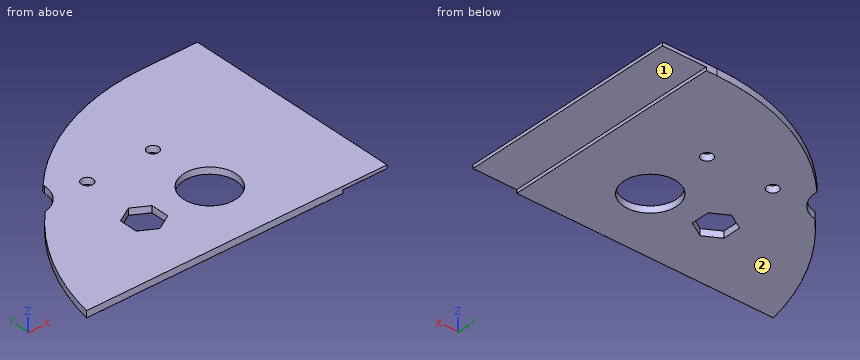
from build123d import *

# Parameters (mm, degrees)
F1_DEPTH  = 3
F3_DEPTH  = 25
F4_R      = 5
F5_R      = 12
F5_R_2    = 2.65
F6_DEPTH  = 25
F7_W      = 78
F7_H      = 55.5
F7_R      = 2
F8_DEPTH  = 25
F9_R      = 8.15
F10_DEPTH = 25
F12_W     = 300.7349916597
F12_H     = 105.2985801398
F13_DEPTH = 25
F14_W     = 20
F14_H     = 100
F15_DEPTH = 1.5
F17_DEPTH = 25
F19_DEPTH = 3


with BuildPart() as f1:
    # F0 (on Top) → F1 (new body)
    with BuildSketch(Plane.XY):
        with BuildLine():
            Line((-197.8147600734, 20.7911690818), (-202.2340594865, 0))
            Line((-202.2340594865, 0), (216.0975214603, 0))
            Line((216.0975214603, 0), (209.2885731253, 20.7911690818))
            ThreePointArc((209.2885731253, 20.7911690818), (167.4870934164, 78.1154778874), (100, 100))
            Line((100, 100), (-100, 100))
            ThreePointArc((-100, 100), (-162.932039105, 77.7145961457), (-197.8147600734, 20.7911690818))
        make_face()
    extrude(amount=F1_DEPTH)

    # F2 (on face) → F3 (cut)
    with BuildSketch(Plane.XY.offset(3)):
        with BuildLine():
            ThreePointArc((1.5842979518, 0), (9.4530988092, 4.1693984068), (12.6, 12.5))
            ThreePointArc((12.6, 12.5), (12.2192388124, 15.5741182224), (11.0999678023, 18.4624420155))
            ThreePointArc((11.0999678023, 18.4624420155), (0, 25.1), (-11.0999678023, 18.4624420155))
            ThreePointArc((-11.0999678023, 18.4624420155), (-11.1999147641, 6.7274867453), (-1.5842979518, 0))
            Line((-1.5842979518, 0), (1.5842979518, 0))
        make_face()
        with BuildLine():
            ThreePointArc((11.0999678023, 18.4624420155), (12.2192388124, 15.5741182224), (12.6, 12.5))
            ThreePointArc((12.6, 12.5), (9.4530988092, 4.1693984068), (1.5842979518, 0))
            Line((1.5842979518, 0), (21.7592636698, 0))
            Line((21.7592636698, 0), (11.0999678023, 18.4624420155))
        make_face()
        with BuildLine():
            ThreePointArc((-1.5842979518, 0), (0, -0.1), (1.5842979518, 0))
            Line((1.5842979518, 0), (-1.5842979518, 0))
        make_face()
        with BuildLine():
            ThreePointArc((-1.5842979518, 0), (-11.1999147641, 6.7274867453), (-11.0999678023, 18.4624420155))
            Line((-11.0999678023, 18.4624420155), (-21.7592636698, 0))
            Line((-21.7592636698, 0), (-1.5842979518, 0))
        make_face()
    extrude(amount=-F3_DEPTH, mode=Mode.SUBTRACT)

    # F4
    f4_edges = [f1.edges().sort_by_distance(p)[0] for p in [
        (-21.759264, 0, 1.5),
        (21.759264, 0, 1.5),
    ]]
    fillet(f4_edges, radius=F4_R)

    # F5 (on face) → F6 (cut)
    with BuildSketch(Plane.XY.offset(3)):
        Polygon((-160, 38.3138438763), (-167.2, 34.1569219382), (-167.2, 25.8430780618), (-160, 21.6861561237), (-152.8, 25.8430780618), (-152.8, 34.1569219382), align=None)
        with Locations((-130, 30)):
            Circle(F5_R)
        with Locations((-130, 60)):
            Circle(F5_R_2)
        with Locations((-160, 60)):
            Circle(F5_R_2)
    extrude(amount=-F6_DEPTH, mode=Mode.SUBTRACT)

    # F7 (on face) → F8 (cut)
    with BuildSketch(Plane.XY.offset(3)):
        with Locations((0, 57.75)):
            Rectangle(F7_W, F7_H)
        with Locations((-42.6313167033, 28.25)):
            Circle(F7_R)
        with Locations((-42.6313167033, 87.25)):
            Circle(F7_R)
        with Locations((42.3686832967, 87.25)):
            Circle(F7_R)
        with Locations((42.3686832967, 28.25)):
            Circle(F7_R)
    extrude(amount=-F8_DEPTH, mode=Mode.SUBTRACT)

    # F9 (on face) → F10 (cut)
    with BuildSketch(Plane.XY.offset(3)):
        with Locations((115, 30)):
            Circle(F9_R)
    extrude(amount=-F10_DEPTH, mode=Mode.SUBTRACT)

    # F12 (on face) → F13 (cut)
    with BuildSketch(Plane.XY.offset(3)):
        with Locations((75.3674958299, 52.6492900699)):
            Rectangle(F12_W, F12_H)
    extrude(amount=-F13_DEPTH, mode=Mode.SUBTRACT)

    # F14 (on face) → F15 (cut)
    with BuildSketch(Plane(origin=(0, 0, 0), x_dir=(1, 0, 0), z_dir=(0, 0, -1))):
        with Locations((-85, -50)):
            Rectangle(F14_W, F14_H)
    extrude(amount=-F15_DEPTH, mode=Mode.SUBTRACT)

    # F16 (on face) → F17 (cut)
    with BuildSketch(Plane.XY.offset(3)):
        with BuildLine():
            ThreePointArc((-183.2262560087, 55.4381665532), (-175.8146533038, 59.7113164576), (-172.8869867134, 67.75))
            ThreePointArc((-172.8869867134, 67.75), (-172.891816845, 68.0974621682), (-172.9063035068, 68.4446558102))
            ThreePointArc((-172.9063035068, 68.4446558102), (-178.3366850582, 62.1559633028), (-183.2262560087, 55.4381665532))
        make_face()
        with BuildLine():
            ThreePointArc((-183.2262560087, 55.4381665532), (-178.3366850582, 62.1559633028), (-172.9063035068, 68.4446558102))
            ThreePointArc((-172.9063035068, 68.4446558102), (-195.1790723457, 75.5194954128), (-183.2262560087, 55.4381665532))
        make_face()
    extrude(amount=-F17_DEPTH, mode=Mode.SUBTRACT)

    # F18 (on face) → F19 (join)
    with BuildSketch(Plane.XY.offset(3)):
        with BuildLine():
            Line((-183.2262560087, 0), (-183.2262560087, 55.4381665532))
            ThreePointArc((-183.2262560087, 55.4381665532), (-201.7549584248, 29.8250444644), (-212.2340594865, 0))
            Line((-212.2340594865, 0), (-183.2262560087, 0))
        make_face()
    extrude(amount=-F19_DEPTH)


solid = f1.part
Can you work these out from the model? Positions are in its coordinate system, mm. Face numbers are marked on the shaded views. A direction names the side the tool comes from. Give positions to 0.01 mm unless a question says otherwise; leave off trailing zeros. Order: outer loops, then holes, each group sorted by start corner. A loop starts at its lowest first (then second) coordinate and runs counter-clockwise, first axis right, second up. Notation, with made-up numbers: M 33.5,76.25 L 72.5,76.25 A28 ccw 72.5,112.25 Z; hole C -27.75,-20.75 d9. An arc over 180 degrees is marked long. Use a Markdown table: item, result. Add a question column.
Item 1: Suppose I cut it at A-A (z = 2). List the corners of the cut face in (x, y) for me.
Item 2: Will these pins go through, and if not, where does the flat tip stop? pin 1 (10 mm diameter, centred on x = -83, y = 58.5, fed in from -Z); pin 2 (4 mm diameter, centred on x = -160, y = 60, fed in from +Z); pin 3 (0.8 mm diameter, centred on y = 70, z = 1, fed in from +X); pin 4 (0.9 mm diameter, centred on y = 28, z = 1.5, fed in from -X).
Item 3: Suppose I cut it at D-D (y = 40). List the corners of the cut face in (x, z) for me.
Item 4: Suppose I cut it at B-B (y = 60). List the corners of the cut face in (x, z) for me.
Item 5: Suppose I cut it at C-C (x = -130). List the corners of the cut face in (y, z) for me.
Item 6: If I drill on L1, parallel to X at y = 34.5, z = 2.6; L2, parallel to Y at x = -130, z = 1.7; L3, parallel to Y at x = -160, z = 0.9, over which ranges is the centre line in solid material (lowest first)? Write a range as [from, to].
Item 7: For the marked faces 1 and 2, which set-ups out of +Z, -Z, +X, -X, +Y, -Y let a thin tool reach every point of the face, with its end or its side?
Answer sheet:
| question | item | result |
|---|---|---|
| 1 | outline | M -212.23,0 L -75,0 L -75,100 L -100,100 A100 ccw -172.91,68.44 A12.5 cw -183.23,55.44 A110 ccw Z; hole M -167.2,25.84 L -160,21.69 L -152.8,25.84 L -152.8,34.16 L -160,38.31 L -167.2,34.16 Z; hole C -160,60 d5.3; hole C -130,30 d24; hole C -130,60 d5.3 |
| 2 | pin 1 | stops at z = 1.5 |
| 2 | pin 2 | passes through |
| 2 | pin 3 | stops at x = -95 |
| 2 | pin 4 | stops at x = -202.91 |
| 3 | outline | M -195.71,0 L -136.63,0 L -136.63,3 L -195.71,3 Z; M -123.37,0 L -95,0 L -95,1.5 L -75,1.5 L -75,3 L -123.37,3 Z |
| 4 | outline | M -175.58,0 L -162.65,0 L -162.65,3 L -175.58,3 Z; M -157.35,0 L -132.65,0 L -132.65,3 L -157.35,3 Z; M -127.35,0 L -95,0 L -95,1.5 L -75,1.5 L -75,3 L -127.35,3 Z |
| 5 | outline | M 0,0 L 18,0 L 18,3 L 0,3 Z; M 42,0 L 57.35,0 L 57.35,3 L 42,3 Z; M 62.65,0 L 95.39,0 L 95.39,3 L 62.65,3 Z |
| 6 | L1 | x = [-199.16, -166.61], [-153.39, -141.12], [-118.88, -75] |
| 6 | L2 | y = [0, 18], [42, 57.35], [62.65, 95.39] |
| 6 | L3 | y = [0, 21.69], [38.31, 57.35], [62.65, 80] |
| 7 | face 1 | -Z, +X, +Y, -Y |
| 7 | face 2 | -Z, +X, -X, +Y, -Y |
